from build123d import *

# Parameters (mm, degrees)
SKETCH9_W           = 1200
SKETCH9_H           = 600
BOSS_EXTRUDE4_DEPTH = 20
SKETCH10_W          = 20
SKETCH10_H          = 580
BOSS_EXTRUDE6_DEPTH = 38
SKETCH11_W          = 20
SKETCH11_H          = 38
BOSS_EXTRUDE7_DEPTH = 760


with BuildPart() as part:
    # Sketch9 → Boss-Extrude4 (new body)
    with BuildSketch(Plane(origin=(0, 0, 0), x_dir=(1, 0, 0), z_dir=(0, 1, 0))):
        with Locations((600, 300)):
            Rectangle(SKETCH9_W, SKETCH9_H)
    extrude(amount=BOSS_EXTRUDE4_DEPTH)

    # Sketch10 → Boss-Extrude6 (add)
    with BuildSketch(Plane(origin=(0, 20, 0), x_dir=(1, 0, 0), z_dir=(0, 1, 0))):
        with Locations((20, 300)):
            Rectangle(SKETCH10_W, SKETCH10_H)
        with Locations((1180, 300)):
            Rectangle(SKETCH10_W, SKETCH10_H)
    extrude(amount=BOSS_EXTRUDE6_DEPTH)

    # Sketch11 → Boss-Extrude7 (add)
    with BuildSketch(Plane(origin=(0, 58, 0), x_dir=(1, 0, 0), z_dir=(0, 1, 0))):
        with Locations((20, 571)):
            Rectangle(SKETCH11_W, SKETCH11_H)
        with Locations((20, 29)):
            Rectangle(SKETCH11_W, SKETCH11_H)
        with Locations((1180, 29)):
            Rectangle(SKETCH11_W, SKETCH11_H)
        with Locations((1180, 571)):
            Rectangle(SKETCH11_W, SKETCH11_H)
    extrude(amount=BOSS_EXTRUDE7_DEPTH)


solid = part.part
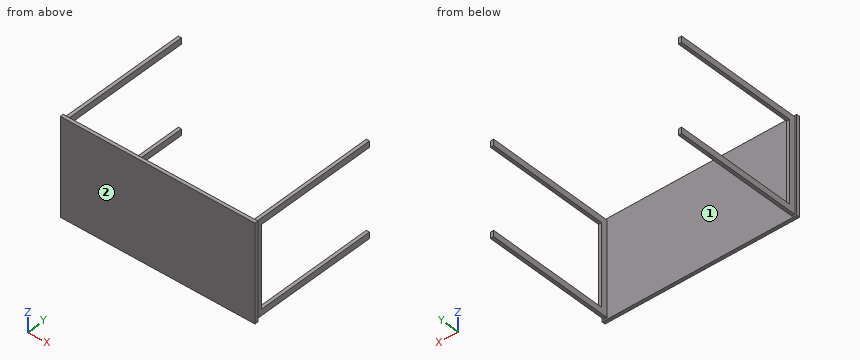
Geometry: final body of the model. Coordinates: model frame, mm. Face numbers are marked on the shaded views. Coordinates: 2 decimals unless noted, no trailing zeros. Loops run counter-clockwise (first coordinate to the right, second up) from the corner with the lowest first, then second, coordinate; pieces in that order, holes last. Notation, with made-up numbers: M 53,-33.75 L 60,-33.75 A13 ccw 60,-17.75 Z; hole C 42.5,65 d7. An arc over 180 degrees is marked long. One line per item, written item: value. Start each with the question number.
1) Cut plane C-C (x = 969). Return loops of the section in (y, z), then the cut area to 3 significant figures.
2) Pin query (flat end, axial travel): P1, Ø4, axis at x = 825, z = -454, coming from the +Y side; P2, Ø6, axis at x = 1180.5, y = 595, coming from the -Z side; P3, Ø22, axis at x = 1185, z = -352.5, coming from the +Y side. Return the tip coordinate at first contact, or that it passes through.
3) Material intervals for L1, parallel to X at y = 233.5, z = -574.5; L2, parallel to Y at x = 768, z = -60, sorted ascending. Write a range as from..to.
4) Draft query along X for the marked faces 1 and 2. Return one class per face: released by +X, released by -X, zero draft, split by the parting line, or undercut.
5) Cut plane A-A (y = 195.5). Return loops of the section in (x, z).
6) Cut plane B-B (z = -455). Return loops of the section in (x, y).
Evaluation:
1. outline: M 0,-600 L 20,-600 L 20,0 L 0,0 Z
1. area: 12,000 mm^2
2. P1: y = 20
2. P2: z = -590
2. P3: y = 58
3. L1: 10..30, 1170..1190
3. L2: 0..20
4. face 1: undercut
4. face 2: zero draft
5. outline: M 10,-590 L 30,-590 L 30,-552 L 10,-552 Z; M 10,-48 L 30,-48 L 30,-10 L 10,-10 Z; M 1170,-590 L 1190,-590 L 1190,-552 L 1170,-552 Z; M 1170,-48 L 1190,-48 L 1190,-10 L 1170,-10 Z
6. outline: M 0,0 L 1200,0 L 1200,20 L 1190,20 L 1190,58 L 1170,58 L 1170,20 L 30,20 L 30,58 L 10,58 L 10,20 L 0,20 Z
